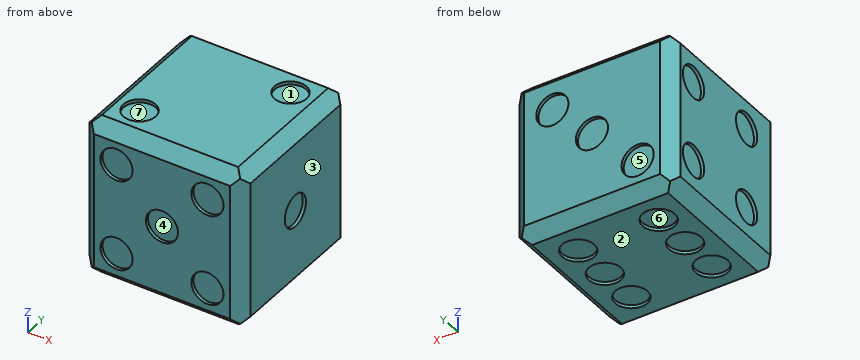
from build123d import *

# Parameters (mm, degrees)
SKETCH1_W           = 127
SKETCH1_H           = 127
CUBE_DEPTH          = 127
SKETCH1_2_W         = 127
SKETCH1_2_H         = 127
BOSS_EXTRUDE2_DEPTH = 127
SKETCH4_R           = 12.7
F_6_DOT_CUT_DEPTH   = 2.54
SKETCH9_R           = 12.7
F_4_DOT_CUT_DEPTH   = 2.54
SKETCH10_R          = 12.7
F_3_DOT_CUT_DEPTH   = 2.54
F_5_DOT_START       = -2.54
SKETCH11_R          = 12.7
F_5_DOT_CUT_DEPTH   = 2.54
SKETCH12_R          = 12.7
F_1_DOT_CUT_DEPTH   = 2.54
SKETCH13_R          = 12.7
F_2_DOT_CUT_DEPTH   = 2.54
CUT_EXTRUDE7_REACH  = 221.97
CUT_EXTRUDE8_REACH  = 221.97
CUT_EXTRUDE9_REACH  = 221.97


with BuildPart() as part:
    # Sketch1 → Cube (new body)
    with BuildSketch(Plane.XY):
        with Locations((63.5, 63.5)):
            Rectangle(SKETCH1_W, SKETCH1_H)
    extrude(amount=CUBE_DEPTH)

    # Sketch1_2 → Boss-Extrude2 (add)
    with BuildSketch(Plane.XY):
        with Locations((63.5, 63.5)):
            Rectangle(SKETCH1_2_W, SKETCH1_2_H)
    extrude(amount=BOSS_EXTRUDE2_DEPTH)

    # Sketch4 → 6-dot cut (cut)
    with BuildSketch(Plane(origin=(0, 0, 0), x_dir=(-1, 0, 0), z_dir=(0, 0, -1))):
        with Locations((-31.75, 63.5)):
            Circle(SKETCH4_R)
        with Locations((-31.75, 31.75)):
            Circle(SKETCH4_R)
        with Locations((-31.75, 95.25)):
            Circle(SKETCH4_R)
        with Locations(Location((-95.25, 31.75, 0), (0, 0, 180))):
            Circle(SKETCH4_R)
        with Locations(Location((-95.25, 63.5, 0), (0, 0, 180))):
            Circle(SKETCH4_R)
        with Locations(Location((-95.25, 95.25, 0), (0, 0, 180))):
            Circle(SKETCH4_R)
    extrude(amount=-F_6_DOT_CUT_DEPTH, mode=Mode.SUBTRACT)

    # Sketch9 → 4-dot cut (cut)
    with BuildSketch(Plane.ZY):
        with Locations(Location((95.25, 101.6, 0), (0, 0, 270))):
            Circle(SKETCH9_R)
        with Locations(Location((95.25, 38.1, 0), (0, 0, 270))):
            Circle(SKETCH9_R)
        with Locations(Location((31.75, 38.1, 0), (0, 0, 90))):
            Circle(SKETCH9_R)
        with Locations(Location((31.75, 101.6, 0), (0, 0, 90))):
            Circle(SKETCH9_R)
    extrude(amount=-F_4_DOT_CUT_DEPTH, mode=Mode.SUBTRACT)

    # Sketch10 → 3-dot cut (cut)
    with BuildSketch(Plane(origin=(0, 127, 0), x_dir=(1, 0, 0), z_dir=(0, 1, 0))):
        with Locations(Location((63.5, -63.5, 0), (0, 0, 270))):
            Circle(SKETCH10_R)
        with Locations(Location((27.403839575, -27.75496954, 0), (0, 0, 270))):
            Circle(SKETCH10_R)
        with Locations(Location((94.798796898, -94.988870563, 0), (0, 0, 270))):
            Circle(SKETCH10_R)
    extrude(amount=-F_3_DOT_CUT_DEPTH, mode=Mode.SUBTRACT)

    # Sketch11 → 5-dot cut (cut)
    with BuildSketch(Plane.XZ.offset(F_5_DOT_START)):
        with Locations(Location((63.5, 63.5, 0), (0, 0, 90))):
            Circle(SKETCH11_R)
        with Locations(Location((27.578975516, 27.578975516, 0), (0, 0, 270))):
            Circle(SKETCH11_R)
        with Locations(Location((99.421024484, 99.421024484, 0), (0, 0, 270))):
            Circle(SKETCH11_R)
        with Locations(Location((27.578975516, 99.421024484, 0), (0, 0, 270))):
            Circle(SKETCH11_R)
        with Locations(Location((99.421024484, 27.578975516, 0), (0, 0, 270))):
            Circle(SKETCH11_R)
    extrude(amount=F_5_DOT_CUT_DEPTH, mode=Mode.SUBTRACT)

    # Sketch12 → 1-dot cut (cut)
    with BuildSketch(Plane(origin=(127, 0, 0), x_dir=(0, 0, -1), z_dir=(1, 0, 0))):
        with Locations(Location((-63.5, 63.5, 0), (0, 0, 90))):
            Circle(SKETCH12_R)
    extrude(amount=-F_1_DOT_CUT_DEPTH, mode=Mode.SUBTRACT)

    # Sketch13 → 2-dot cut (cut)
    with BuildSketch(Plane.XY.offset(127)):
        with Locations((27.578975516, 27.578975516)):
            Circle(SKETCH13_R)
        with Locations((99.421024484, 99.421024484)):
            Circle(SKETCH13_R)
    extrude(amount=-F_2_DOT_CUT_DEPTH, mode=Mode.SUBTRACT)

    # Sketch16 → Cut-Extrude7 (cut, up to next)
    with BuildSketch(Plane.ZY, mode=Mode.PRIVATE) as cut_extrude7_sk1:
        Polygon((0, 127), (9.652, 127), (0, 117.348), align=None)
    cut_extrude7_tool1 = extrude(cut_extrude7_sk1.sketch, amount=-CUT_EXTRUDE7_REACH, mode=Mode.PRIVATE) & part.part
    # Sketch16 → Cut-Extrude7 (cut, up to next)
    with BuildSketch(Plane.ZY, mode=Mode.PRIVATE) as cut_extrude7_sk2:
        Polygon((117.348, 127), (127, 117.348), (127, 127), align=None)
    cut_extrude7_tool2 = extrude(cut_extrude7_sk2.sketch, amount=-CUT_EXTRUDE7_REACH, mode=Mode.PRIVATE) & part.part
    # Sketch16 → Cut-Extrude7 (cut, up to next)
    with BuildSketch(Plane.ZY, mode=Mode.PRIVATE) as cut_extrude7_sk3:
        Polygon((127, 0), (117.348, 0), (127, 9.652), align=None)
    cut_extrude7_tool3 = extrude(cut_extrude7_sk3.sketch, amount=-CUT_EXTRUDE7_REACH, mode=Mode.PRIVATE) & part.part
    # Sketch16 → Cut-Extrude7 (cut, up to next)
    with BuildSketch(Plane.ZY, mode=Mode.PRIVATE) as cut_extrude7_sk4:
        Polygon((9.652, 0), (0, 9.652), (0, 0), align=None)
    cut_extrude7_tool4 = extrude(cut_extrude7_sk4.sketch, amount=-CUT_EXTRUDE7_REACH, mode=Mode.PRIVATE) & part.part
    add(cut_extrude7_tool1.solids().sort_by_distance((0, 123.782667, 3.217333))[0], mode=Mode.SUBTRACT)
    add(cut_extrude7_tool2.solids().sort_by_distance((0, 123.782667, 123.782667))[0], mode=Mode.SUBTRACT)
    add(cut_extrude7_tool3.solids().sort_by_distance((0, 3.217333, 123.782667))[0], mode=Mode.SUBTRACT)
    add(cut_extrude7_tool4.solids().sort_by_distance((0, 3.217333, 3.217333))[0], mode=Mode.SUBTRACT)

    # Sketch17 → Cut-Extrude8 (cut, up to next)
    with BuildSketch(Plane.XY.offset(127), mode=Mode.PRIVATE) as cut_extrude8_sk1:
        Polygon((9.652, 127), (0, 127), (0, 117.348), align=None)
    cut_extrude8_tool1 = extrude(cut_extrude8_sk1.sketch, amount=-CUT_EXTRUDE8_REACH, mode=Mode.PRIVATE) & part.part
    # Sketch17 → Cut-Extrude8 (cut, up to next)
    with BuildSketch(Plane.XY.offset(127), mode=Mode.PRIVATE) as cut_extrude8_sk2:
        Polygon((117.348, 127), (127, 117.348), (127, 127), align=None)
    cut_extrude8_tool2 = extrude(cut_extrude8_sk2.sketch, amount=-CUT_EXTRUDE8_REACH, mode=Mode.PRIVATE) & part.part
    # Sketch17 → Cut-Extrude8 (cut, up to next)
    with BuildSketch(Plane.XY.offset(127), mode=Mode.PRIVATE) as cut_extrude8_sk3:
        Polygon((117.348, 0), (127, 0), (127, 9.652), align=None)
    cut_extrude8_tool3 = extrude(cut_extrude8_sk3.sketch, amount=-CUT_EXTRUDE8_REACH, mode=Mode.PRIVATE) & part.part
    # Sketch17 → Cut-Extrude8 (cut, up to next)
    with BuildSketch(Plane.XY.offset(127), mode=Mode.PRIVATE) as cut_extrude8_sk4:
        Polygon((9.652, 0), (0, 0), (0, 9.652), align=None)
    cut_extrude8_tool4 = extrude(cut_extrude8_sk4.sketch, amount=-CUT_EXTRUDE8_REACH, mode=Mode.PRIVATE) & part.part
    add(cut_extrude8_tool1.solids().sort_by_distance((3.217333, 123.782667, 127))[0], mode=Mode.SUBTRACT)
    add(cut_extrude8_tool2.solids().sort_by_distance((123.782667, 123.782667, 127))[0], mode=Mode.SUBTRACT)
    add(cut_extrude8_tool3.solids().sort_by_distance((123.782667, 3.217333, 127))[0], mode=Mode.SUBTRACT)
    add(cut_extrude8_tool4.solids().sort_by_distance((3.217333, 3.217333, 127))[0], mode=Mode.SUBTRACT)

    # Sketch18 → Cut-Extrude9 (cut, up to next)
    with BuildSketch(Plane(origin=(0, 127, 0), x_dir=(1, 0, 0), z_dir=(0, 1, 0)), mode=Mode.PRIVATE) as cut_extrude9_sk1:
        Polygon((0, 0), (9.652, 0), (0, -9.652), align=None)
    cut_extrude9_tool1 = extrude(cut_extrude9_sk1.sketch, amount=-CUT_EXTRUDE9_REACH, mode=Mode.PRIVATE) & part.part
    # Sketch18 → Cut-Extrude9 (cut, up to next)
    with BuildSketch(Plane(origin=(0, 127, 0), x_dir=(1, 0, 0), z_dir=(0, 1, 0)), mode=Mode.PRIVATE) as cut_extrude9_sk2:
        Polygon((117.348, 0), (127, -9.652), (127, 0), align=None)
    cut_extrude9_tool2 = extrude(cut_extrude9_sk2.sketch, amount=-CUT_EXTRUDE9_REACH, mode=Mode.PRIVATE) & part.part
    # Sketch18 → Cut-Extrude9 (cut, up to next)
    with BuildSketch(Plane(origin=(0, 127, 0), x_dir=(1, 0, 0), z_dir=(0, 1, 0)), mode=Mode.PRIVATE) as cut_extrude9_sk3:
        Polygon((127, -127), (117.348, -127), (127, -117.348), align=None)
    cut_extrude9_tool3 = extrude(cut_extrude9_sk3.sketch, amount=-CUT_EXTRUDE9_REACH, mode=Mode.PRIVATE) & part.part
    # Sketch18 → Cut-Extrude9 (cut, up to next)
    with BuildSketch(Plane(origin=(0, 127, 0), x_dir=(1, 0, 0), z_dir=(0, 1, 0)), mode=Mode.PRIVATE) as cut_extrude9_sk4:
        Polygon((9.652, -127), (0, -117.348), (0, -127), align=None)
    cut_extrude9_tool4 = extrude(cut_extrude9_sk4.sketch, amount=-CUT_EXTRUDE9_REACH, mode=Mode.PRIVATE) & part.part
    add(cut_extrude9_tool1.solids().sort_by_distance((3.217333, 127, 3.217333))[0], mode=Mode.SUBTRACT)
    add(cut_extrude9_tool2.solids().sort_by_distance((123.782667, 127, 3.217333))[0], mode=Mode.SUBTRACT)
    add(cut_extrude9_tool3.solids().sort_by_distance((123.782667, 127, 123.782667))[0], mode=Mode.SUBTRACT)
    add(cut_extrude9_tool4.solids().sort_by_distance((3.217333, 127, 123.782667))[0], mode=Mode.SUBTRACT)


solid = part.part
Verification items for the finished model (mm, model axes). Face numbers are marked on the shaded views. A direction names the side the tool comes from. Coordinates: 2 decimals unless noted, no trailing zeros. Order: outer loops, then holes, each group sorted by start corner. A loop starts at its lowest first (then second) coordinate and runs counter-clockwise, first axis right, second up.
Item 1: Material ranges on L1, parallel to Y at x = 31, z = 1; L2, parallel to X at y = 110.5, z = 100.5; L3, parallel to Z at x = 126, y = 63, recorded low to high.
Filled in:
L1: y = 8.65 to 19.07, 44.43 to 50.82, 76.18 to 82.57, 107.93 to 118.35
L2: x = 2.54 to 127
L3: z = 8.65 to 50.81, 76.19 to 118.35
Item 2: Section check A-A, the plane x = 63.5. Enter the section's corners in (y, z).
Filled in:
outline: (0, 9.65) - (9.65, 0) - (117.35, 0) - (127, 9.65) - (127, 50.8) - (124.46, 50.8) - (124.46, 76.2) - (127, 76.2) - (127, 117.35) - (117.35, 127) - (9.65, 127) - (0, 117.35) - (0, 76.2) - (2.54, 76.2) - (2.54, 50.8) - (0, 50.8) - close
Item 3: Access from +Z, -Z, +X, -X, +Y, -Y to the whole of each face (thin tool, end or side, straight path). Record for the marked faces 4, 5, 6 and 7.
Filled in:
face 4: -Y
face 5: +Y
face 6: -Z
face 7: +Z
Item 4: Release check for a two-part mould opening along X. For the marked faces 1, 2 and 3 record: +X half, -X half, draft (parallel to the pull), parting line (faces both ways), or undercut.
Filled in:
face 1: undercut
face 2: draft
face 3: +X half
Item 5: Section check B-B, the plane z = 63.5. Enter the section's corners in (x, y).
Filled in:
outline: (0, 9.65) - (9.65, 0) - (50.8, 0) - (50.8, 2.54) - (76.2, 2.54) - (76.2, 0) - (117.35, 0) - (127, 9.65) - (127, 50.8) - (124.46, 50.8) - (124.46, 76.2) - (127, 76.2) - (127, 117.35) - (117.35, 127) - (76.2, 127) - (76.2, 124.46) - (50.8, 124.46) - (50.8, 127) - (9.65, 127) - (0, 117.35) - close
Item 6: Section check C-C, the plane y = 38.1. Enter the section's corners in (x, z), then the cut area to 3 significant figures.
Filled in:
outline: (0, 9.65) - (9.65, 0) - (20.75, 0) - (20.75, 2.54) - (42.75, 2.54) - (42.75, 0) - (84.25, 0) - (84.25, 2.54) - (106.25, 2.54) - (106.25, 0) - (117.35, 0) - (127, 9.65) - (127, 117.35) - (117.35, 127) - (34.69, 127) - (34.69, 124.46) - (20.47, 124.46) - (20.47, 127) - (9.65, 127) - (0, 117.35) - (0, 107.95) - (2.54, 107.95) - (2.54, 82.55) - (0, 82.55) - (0, 44.45) - (2.54, 44.45) - (2.54, 19.05) - (0, 19.05) - close
area: 15,700 mm2
Item 7: Section check D-D, the plane z = 25.5. Enter the section's corners in (x, y).
Filled in:
outline: (0, 9.65) - (9.65, 0) - (15.05, 0) - (15.05, 2.54) - (40.11, 2.54) - (40.11, 0) - (86.89, 0) - (86.89, 2.54) - (111.95, 2.54) - (111.95, 0) - (117.35, 0) - (127, 9.65) - (127, 117.35) - (117.35, 127) - (39.9, 127) - (39.9, 124.46) - (14.91, 124.46) - (14.91, 127) - (9.65, 127) - (0, 117.35) - (0, 112.66) - (2.54, 112.66) - (2.54, 90.54) - (0, 90.54) - (0, 49.16) - (2.54, 49.16) - (2.54, 27.04) - (0, 27.04) - close
Item 8: Depth check by flat-ended pin: pin 1 (1 mm diameter, centred on x = 70.5, z = 58.5, fed in from -Y); pin 2 (7.5 mm diameter, centred on x = 94, z = 91, fed in from +Y); pin 3 (12.5 mm diameter, centred on x = 37.5, y = 32, fed in from -Z). Enter the tip coordinate at first touch or a pass-through.
Filled in:
pin 1: stops at y = 2.54
pin 2: stops at y = 124.46
pin 3: stops at z = 2.54
